from build123d import *

# Parameters (mm, degrees)
F0_R     = 50
F1_DEPTH = 46
F3_DEPTH = 15
F4_W     = 19.177
F4_H     = 19.177
F5_DEPTH = 46.001
F7_R     = 2
F8_DEPTH = 40.4115


with BuildPart() as f1:
    # F0 (on Top) → F1 (new body)
    with BuildSketch(Plane.XY):
        Circle(F0_R)
    extrude(amount=F1_DEPTH)

    # F2 (on face) → F3 (cut)
    with BuildSketch(Plane.XY.offset(46)):
        with BuildLine():
            ThreePointArc((-4.75, 42.485292), (-6.468315, 43.969319), (-7.686451, 42.053311))
            ThreePointArc((-7.686451, 42.053311), (-30.228815, 30.228815), (-42.053311, 7.686451))
            ThreePointArc((-42.053311, 7.686451), (-43.969319, 6.468315), (-42.485292, 4.75))
            Line((-42.485292, 4.75), (-38, 4.75))
            ThreePointArc((-38, 4.75), (-33.25, 0), (-38, -4.75))
            Line((-38, -4.75), (-42.485292, -4.75))
            ThreePointArc((-42.485292, -4.75), (-43.969319, -6.468315), (-42.053311, -7.686451))
            ThreePointArc((-42.053311, -7.686451), (-30.228815, -30.228815), (-7.686451, -42.053311))
            ThreePointArc((-7.686451, -42.053311), (-6.468315, -43.969319), (-4.75, -42.485292))
            Line((-4.75, -42.485292), (-4.75, -38))
            ThreePointArc((-4.75, -38), (0, -33.25), (4.75, -38))
            Line((4.75, -38), (4.75, -42.485292))
            ThreePointArc((4.75, -42.485292), (6.468315, -43.969319), (7.686451, -42.053311))
            ThreePointArc((7.686451, -42.053311), (30.228815, -30.228815), (42.053311, -7.686451))
            ThreePointArc((42.053311, -7.686451), (43.969319, -6.468315), (42.485292, -4.75))
            Line((42.485292, -4.75), (38, -4.75))
            ThreePointArc((38, -4.75), (33.25, 0), (38, 4.75))
            Line((38, 4.75), (42.485292, 4.75))
            ThreePointArc((42.485292, 4.75), (43.969319, 6.468315), (42.053311, 7.686451))
            ThreePointArc((42.053311, 7.686451), (30.228815, 30.228815), (7.686451, 42.053311))
            ThreePointArc((7.686451, 42.053311), (6.468315, 43.969319), (4.75, 42.485292))
            Line((4.75, 42.485292), (4.75, 38))
            ThreePointArc((4.75, 38), (0, 33.25), (-4.75, 38))
            Line((-4.75, 38), (-4.75, 42.485292))
        make_face()
    extrude(amount=-F3_DEPTH, mode=Mode.SUBTRACT)

    # F4 (on face) → F5 (cut, through all)
    with BuildSketch(Plane(origin=(0, 0, 0), x_dir=(1, 0, 0), z_dir=(0, 0, -1))):
        Rectangle(F4_W, F4_H)
    extrude(amount=-F5_DEPTH, mode=Mode.SUBTRACT)

    # F7 (on offset) → F8 (cut, through all)
    with BuildSketch(Plane.YZ.offset(50)):
        with Locations((0, 9.5)):
            Circle(F7_R)
    extrude(amount=-F8_DEPTH, mode=Mode.SUBTRACT)


solid = f1.part
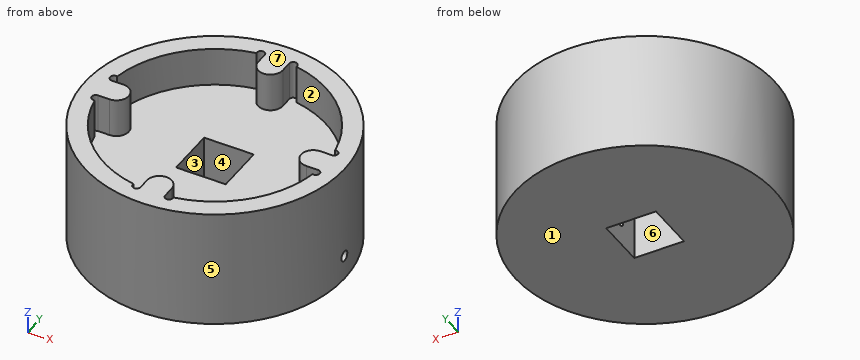
Geometry check sheet. Reference: the model listing, model coordinates, mm. Face numbers are marked on the shaded views. A direction names the side the tool comes from. Round coordinates to 2 decimals unless told otherwise and drop trailing zeros. Loops run counter-clockwise (first coordinate to the right, second up) from the corner with the lowest first, then second, coordinate; pieces in that order, holes last. Notation, with made-up numbers: (39.25, -9.75) -> (74.25, -9.75) arc R24 cw to (74.25, 26.25) -> close; hole circle Ø5 at (26, 23.25). An arc over 180 degrees is marked (long way). Answer as a JSON object with one key per item and string values. Group by question number.
Item 1: Cross-section at B-B, the plane x = 0. Record the cut outline in (y, z).
Item 2: Thickness scan on line 1 along Y through (x, z) = (-35.5, 40); line 2 along Z through (x, y) = (45, 0); line 3 along Z through (x, y) = (-10.5, -17). Record the ranges inside material, lowest first.
Item 3: Cross-section at C-C, the plane y = 6.25. Record the cut outline in (x, z).
Item 4: Cross-section at D-D, the plane z = 22. Record the cut outline in (x, y).
Item 5: Depth check by flat-ended pin: pin 1 Ø1.5 at (x, y) = (-31, 0) entering from -Z; pin 2 Ø6 at (y, z) = (-11.5, 24.5) entering from +X; pin 3 Ø5 at (y, z) = (-39, 39.5) entering from -X; pin 4 Ø1 at (y, z) = (10, 11) entering from -X. Enter the tip coordinate at first touch or a pass-through.
Item 6: Set-up check for the marked faces 1, 2 and 3: record each of +Z, -Z, +X, -X, +Y, -Y from which the full face is reachable in a straight line by a thin tool's end or side.
Item 7: Release check for a two-part mould opening along X. For the marked faces 4, 5, 6 and 7 record: pulls with the +X half, pulls with the -X half, needs draft (parallel to the pull), parting line crosses it, or undercut.
Item 8: Cross-section at A-A, the plane z = 34. Record the cut outline in (x, y).
Determined:
{
 "1": {"outline": "(-50, 0) -> (-9.59, 0) -> (-9.59, 31) -> (-33.25, 31) -> (-33.25, 46) -> (-50, 46) -> close; (9.59, 0) -> (50, 0) -> (50, 46) -> (33.25, 46) -> (33.25, 31) -> (9.59, 31) -> close"},
 "2": {"line 1": "y = -35.21 to -23.82, -4.04 to 4.04, 23.82 to 35.21", "line 2": "z = 0 to 7.5, 11.5 to 46", "line 3": "z = 0 to 31"},
 "3": {"outline": "(-49.61, 0) -> (-9.59, 0) -> (-9.59, 31) -> (-43.99, 31) -> (-43.99, 46) -> (-49.61, 46) -> close; (9.59, 0) -> (49.61, 0) -> (49.61, 46) -> (43.99, 46) -> (43.99, 31) -> (9.59, 31) -> close"},
 "4": {"outline": "circle Ø100 at (0, 0); hole (-9.59, -9.59) -> (9.59, -9.59) -> (9.59, 9.59) -> (-9.59, 9.59) -> close"},
 "5": {"pin 1": "stops at z = 0", "pin 2": "stops at x = 49.27", "pin 3": "stops at x = -34.17", "pin 4": "stops at x = -49.09"},
 "6": {"face 1": "-Z, +X, -X, +Y, -Y", "face 2": "+Z", "face 3": "+Z, -Z"},
 "7": {"face 4": "undercut", "face 5": "parting line crosses it", "face 6": "undercut", "face 7": "needs draft"},
 "8": {"outline": "circle Ø100 at (0, 0); hole (-42.49, -4.75) arc R1.5 ccw (long way) to (-42.05, -7.69) arc R42.75 ccw to (-7.69, -42.05) arc R1.5 ccw (long way) to (-4.75, -42.49) -> (-4.75, -38) arc R4.75 cw to (4.75, -38) -> (4.75, -42.49) arc R1.5 ccw (long way) to (7.69, -42.05) arc R42.75 ccw to (42.05, -7.69) arc R1.5 ccw (long way) to (42.49, -4.75) -> (38, -4.75) arc R4.75 cw to (38, 4.75) -> (42.49, 4.75) arc R1.5 ccw (long way) to (42.05, 7.69) arc R42.75 ccw to (7.69, 42.05) arc R1.5 ccw (long way) to (4.75, 42.49) -> (4.75, 38) arc R4.75 cw to (-4.75, 38) -> (-4.75, 42.49) arc R1.5 ccw (long way) to (-7.69, 42.05) arc R42.75 ccw to (-42.05, 7.69) arc R1.5 ccw (long way) to (-42.49, 4.75) -> (-38, 4.75) arc R4.75 cw to (-38, -4.75) -> close"}
}
